from build123d import *

# Parameters (mm, degrees)
SKETCH1_W           = 38.1
SKETCH1_H           = 38.1
SKETCH1_R           = 11.43
BOSS_EXTRUDE1_DEPTH = 4.7625
SKETCH2_R           = 1.6002
SKETCH2_R_2         = 1.4351
CUT_EXTRUDE1_DEPTH  = 28.358479604
CIRPATTERN1_COUNT   = 4
CHAMFER1_SIZE       = 2.54


with BuildPart() as part:
    # Sketch1 → Boss-Extrude1 (new body)
    with BuildSketch(Plane(origin=(0, 0, 0), x_dir=(1, 0, 0), z_dir=(0, 1, 0))):
        Rectangle(SKETCH1_W, SKETCH1_H)
        with Locations(Location((0, 0, 0), (0, 0, 90))):
            Circle(SKETCH1_R, mode=Mode.SUBTRACT)
    extrude(amount=BOSS_EXTRUDE1_DEPTH)

    # Sketch2 → Cut-Extrude1 (cut, through all)
    with BuildSketch(Plane(origin=(0, 4.7625, 0), x_dir=(1, 0, 0), z_dir=(0, 1, 0))):
        with Locations(Location((0, 13.9954, 0), (0, 0, 270))):
            Circle(SKETCH2_R)
        with Locations(Location((15.24, 15.24, 0), (0, 0, 270))):
            Circle(SKETCH2_R_2)
    cut_extrude1 = extrude(amount=-CUT_EXTRUDE1_DEPTH, mode=Mode.SUBTRACT)

    # CirPattern1: Cut-Extrude1 ×4 about axis
    cirpattern1_axis = Axis((0, 0, 0), (0, 1, 0))
    for i in range(1, CIRPATTERN1_COUNT):
        add(cut_extrude1.rotate(cirpattern1_axis, i * 360 / CIRPATTERN1_COUNT), mode=Mode.SUBTRACT)

    # Chamfer1
    chamfer1_edges = [part.edges().sort_by_distance(p)[0] for p in [
        (19.05, 2.38125, 19.05),
        (-19.05, 2.38125, 19.05),
        (-19.05, 2.38125, -19.05),
        (19.05, 2.38125, -19.05),
    ]]
    chamfer(chamfer1_edges, length=CHAMFER1_SIZE)


solid = part.part
Here's how the part is built. I have some questions about the finished solid (model axes, mm). Give positions to 0.01 mm unless a question says otherwise; leave off trailing zeros. Loops run counter-clockwise (first coordinate to the right, second up) from the corner with the lowest first, then second, coordinate; pieces in that order, holes last. Notation, with made-up numbers: (51.25, -24.75) -> (104.25, -24.75) arc R18 cw to (104.25, 8.25) -> close; hole circle Ø4 at (34.25, 57.25). An arc over 180 degrees is marked (long way). Answer as a JSON object with one key per item and string values. Group by question number.
Item 1: Imagine slicing it at A-A on z = 0. Write out the boundary of the cut face in (x, y).
Item 2: Thinking about a two-plate mould opening in Z: for faces 1 (the cylindrical face through (-0.07, 2.415, 15.594)), 2 (the flat face through (0, 2, 19.05)), 3 (the flat face through (19.05, 2, 0)), which applies, pulls with the +Z half, pulls with the -Z half, needs draft (parallel to the pull), parting line crosses it, or undercut?
Item 3: Imagine slicing it at C-C on x = 0. Write out the boundary of the cut face in (y, z), then the cut area to 3 significant figures.
Item 4: Imagine slicing it at D-D on x = -8. Write out the boundary of the cut face in (y, z).
Item 5: I need wall thicknesses on L1, parallel to X at y = 3.45, z = -16; L2, parallel to Z at x = -8, y = 2.7; L3, parallel to Z at x = -2.5, y = 2.25. Which ranges of each line are inside material? Lowest first, please.
Item 6: Will this pin go through, and if not, where does the flat tip stop? pin 1 (1.7 mm diameter, centred on x = 15.24, z = 15.24, fed in from -Y).
Item 7: Imagine slicing it at B-B on y = 2.95. Give the number of separate pieces and of enclosed holes in the cut face, then the cut area to 3 significant figures.
Answer list:
{
 "1": {"outline": "(-19.05, 0) -> (-15.6, 0) -> (-15.6, 4.76) -> (-19.05, 4.76) -> close; (-12.4, 0) -> (-11.43, 0) -> (-11.43, 4.76) -> (-12.4, 4.76) -> close; (11.43, 0) -> (12.4, 0) -> (12.4, 4.76) -> (11.43, 4.76) -> close; (15.6, 0) -> (19.05, 0) -> (19.05, 4.76) -> (15.6, 4.76) -> close"},
 "2": {"face 1": "undercut", "face 2": "pulls with the +Z half", "face 3": "needs draft"},
 "3": {"outline": "(0, -19.05) -> (4.76, -19.05) -> (4.76, -15.6) -> (0, -15.6) -> close; (0, -12.4) -> (4.76, -12.4) -> (4.76, -11.43) -> (0, -11.43) -> close; (0, 11.43) -> (4.76, 11.43) -> (4.76, 12.4) -> (0, 12.4) -> close; (0, 15.6) -> (4.76, 15.6) -> (4.76, 19.05) -> (0, 19.05) -> close", "area": "42.1 mm2"},
 "4": {"outline": "(0, -19.05) -> (4.76, -19.05) -> (4.76, -8.16) -> (0, -8.16) -> close; (0, 8.16) -> (4.76, 8.16) -> (4.76, 19.05) -> (0, 19.05) -> close"},
 "5": {"L1": "x = -19.05 to -16.46, -14.02 to 14.02, 16.46 to 19.05", "L2": "z = -19.05 to -8.16, 8.16 to 19.05", "L3": "z = -19.05 to -11.15, 11.15 to 19.05"},
 "6": {"pin 1": "passes through"},
 "7": {"separate pieces": "1", "enclosed holes": "9", "area": "970 mm2"}
}
